Could you check a few things on this drawing? It's one solid part, dimensions in mm from its lowest x, y, z. A direction names the side the tool comes from. Give positions to 0.01 mm unless a question says otherwise; leave off trailing zeros. Order: outer loops, then holes, each group sorted by start corner. A loop starts at its lowest first (then second) coordinate and runs counter-clockwise, first axis right, second up.
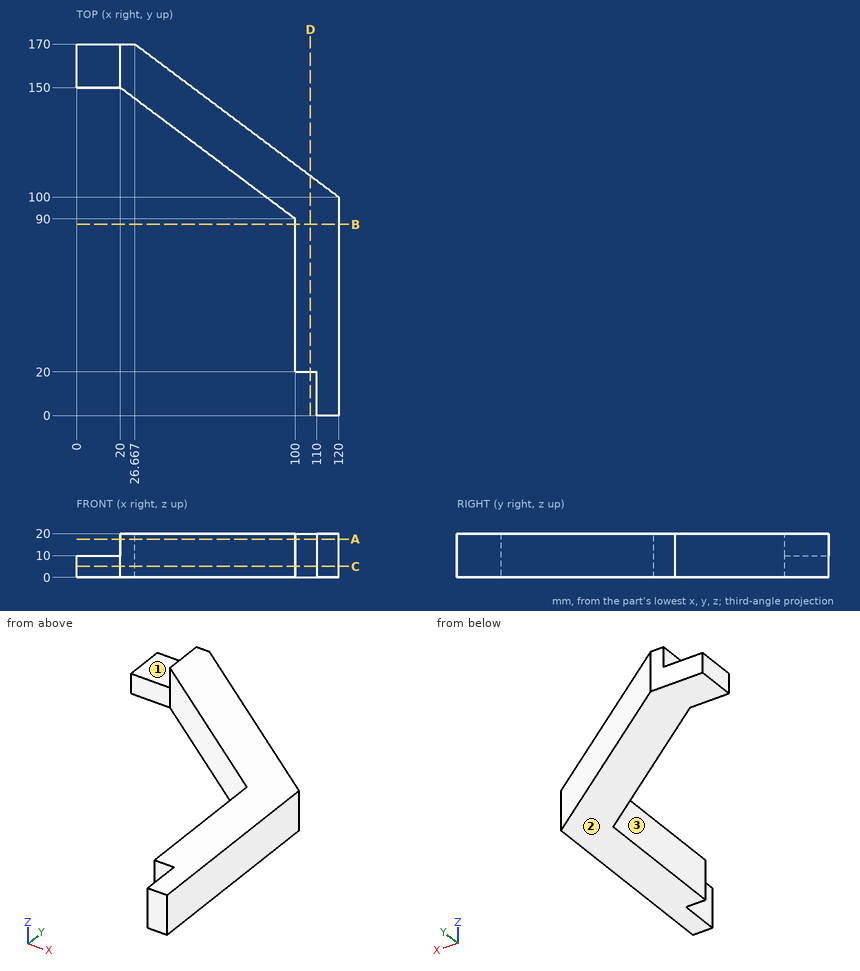
Q1. If we section it at C-C on z = 5: List the corners of the cut face in (x, y) for me.
Filled sheet:
outline: (0, 150) - (20, 150) - (100, 90) - (100, 20) - (110, 20) - (110, 0) - (120, 0) - (120, 100) - (26.67, 170) - (0, 170) - close
Q2. I need wall thicknesses on L1, parallel to X at y = 11, z = 11.25; L2, parallel to X at y = 21, z = 10.25; L3, parallel to Y at x = 25, z = 17. Which ranges of each line are inside material? Lowest first, please.
Filled sheet:
L1: x = 110 to 120
L2: x = 100 to 120
L3: y = 146.25 to 170
Q3. If we section it at B-B on y = 87.5: List the corners of the cut face in (x, z) for me.
Filled sheet:
outline: (100, 0) - (120, 0) - (120, 20) - (100, 20) - close
Q4. For the marked faces 1, 2 and 3, which set-ups out of +Z, -Z, +X, -X, +Y, -Y let a thin tool reach every point of the face, with its end or its side?
Filled sheet:
face 1: +Z, -X, +Y, -Y
face 2: -Z, +X, -X, +Y, -Y
face 3: +Z, -Z, -X, -Y
Q5. If we section it at A-A on z = 17.5: List the corners of the cut face in (x, y) for me.
Filled sheet:
outline: (20, 150) - (100, 90) - (100, 20) - (110, 20) - (110, 0) - (120, 0) - (120, 100) - (26.67, 170) - (20, 170) - close
Q6. I'm going to push flat-ended pins straight in: P1, Ø6, axis at y = 76.5, z = 16.5, coming from the -X side; P2, Ø5, axis at y = 163, z = 17, coming from the -X side; P3, Ø3, axis at x = 92.5, z = 8, coming from the -Y side. Where does each tip first touch, or does it pass through?
Filled sheet:
P1: stops at x = 100
P2: stops at x = 20
P3: stops at y = 94.5
Q7. If we section it at D-D on x = 107: List the corners of the cut face in (y, z) for me, plus the area to 4 significant figures.
Filled sheet:
outline: (20, 0) - (109.75, 0) - (109.75, 20) - (20, 20) - close
area: 1,795 mm2
